from build123d import *

# Parameters (mm, degrees)
SKETCH1_W           = 129
SKETCH1_H           = 7
BOSS_EXTRUDE1_DEPTH = 7
BOSS_EXTRUDE2_START = 0.5
BOSS_EXTRUDE2_DEPTH = 0.5
SKETCH3_W           = 131
SKETCH3_H           = 7
CUT_EXTRUDE4_DEPTH  = 7
CUT_EXTRUDE5_DEPTH  = 7


with BuildPart() as part:
    # Sketch1 → Boss-Extrude1 (new body)
    with BuildSketch(Plane(origin=(0, 0, 0), x_dir=(1, 0, 0), z_dir=(0, 1, 0))):
        with BuildLine():
            Line((-65.5, 5.5), (-65.5, -3.5))
            ThreePointArc((-65.5, -3.5), (0, -56.5), (65.5, -3.5))
            Line((65.5, -3.5), (65.5, 5.5))
            Line((65.5, 5.5), (-65.5, 5.5))
        make_face()
        Rectangle(SKETCH1_W, SKETCH1_H, mode=Mode.SUBTRACT)
    extrude(amount=BOSS_EXTRUDE1_DEPTH)

    # Sketch2 → Boss-Extrude2 (add)
    with BuildSketch(Plane.XZ.offset(BOSS_EXTRUDE2_START)):
        with BuildLine():
            Line((-65.5, -5.5), (65.5, -5.5))
            Line((65.5, -5.5), (65.5, 3.5))
            ThreePointArc((65.5, 3.5), (0, 56.5), (-65.5, 3.5))
            Line((-65.5, 3.5), (-65.5, -5.5))
        make_face()
    extrude(amount=-BOSS_EXTRUDE2_DEPTH)

    # Sketch3 → Cut-Extrude4 (cut)
    with BuildSketch(Plane(origin=(0, 7, 0), x_dir=(1, 0, 0), z_dir=(0, 1, 0))):
        Rectangle(SKETCH3_W, SKETCH3_H)
    extrude(amount=-CUT_EXTRUDE4_DEPTH, mode=Mode.SUBTRACT)

    # Sketch4 → Cut-Extrude5 (cut)
    with BuildSketch(Plane(origin=(0, 7, 0), x_dir=(1, 0, 0), z_dir=(0, 1, 0))):
        with BuildLine():
            Line((58.998041221, -8.5), (-58.998041221, -8.5))
            ThreePointArc((-58.998041221, -8.5), (0, -51.5), (58.998041221, -8.5))
        make_face()
    extrude(amount=-CUT_EXTRUDE5_DEPTH, mode=Mode.SUBTRACT)


solid = part.part
Design review of the part built by this model. Coordinates are the model's own, in mm. A direction names the side the tool comes from. Give positions to 0.01 mm unless a question says otherwise; leave off trailing zeros. Loops run counter-clockwise (first coordinate to the right, second up) from the corner with the lowest first, then second, coordinate; pieces in that order, holes last. Notation, with made-up numbers: (38, 72.5) - (80, 72.5) arc R22 ccw to (80, 82.5) - close; hole circle Ø6 at (-30.75, 86). An arc over 180 degrees is marked (long way). Write item = value, one per line.
1) Tool access review of faces 5 (the face through (65.5, 3, -4)), 6 (the face through (1, 4, 8.5)), 7 (the face through (-1, 4, -3.5)): name each direction out of +Z, -Z, +X, -X, +Y, -Y from which nothing blocks a thin tool from reaching the whole face with its end or side.
Result sheet:
face_5 = +Z, -Z, +X, +Y, -Y
face_6 = +Y
face_7 = +X, -X, +Y
2) Take a section at A-A on y = 4. State the section outline as (x, z) points.
Result sheet:
outline = (-65.5, -5.5) - (65.5, -5.5) - (65.5, -3.5) - (-65.5, -3.5) - close; (-65.5, 3.5) - (65.5, 3.5) arc R66.97 ccw to start; hole (-59, 8.5) - (59, 8.5) arc R61.97 ccw to start
3) Take a section at D-D on x = -41.5. State the section outline as (y, z) points, and give its area (3 significant figures).
Result sheet:
outline = (-0.5, -5.5) - (7, -5.5) - (7, -3.5) - (0, -3.5) - (0, 3.5) - (7, 3.5) - (7, 8.5) - (0, 8.5) - (0, 35.55) - (7, 35.55) - (7, 42.09) - (-0.5, 42.09) - close
area = 119 mm2
4) Clearance check with flat-ended pins moving along their axes: pin 1 Ø1.5 at (x, y) = (48, 4) entering from +Z; pin 2 Ø1.5 at (y, z) = (5, 13) entering from +X; pin 3 Ø1.5 at (y, z) = (5.5, 32.5) entering from +X. State where each tip first meets the part, or that it passes through.
Result sheet:
pin_1 = 36.99
pin_2 = 63
pin_3 = 51.99
5) Take a section at C-C on z = 26.5. State the section outline as (x, y) points.
Result sheet:
outline = (-55.84, -0.5) - (55.84, -0.5) - (55.84, 7) - (49.74, 7) - (49.74, 0) - (-49.74, 0) - (-49.74, 7) - (-55.84, 7) - close
6) To check wall thickness, follow line 1 (Z direction, x = 56, y = 2.5); line 2 (Z direction, x = 32, y = 5); line 3 (Y direction, x = -44, z = -2). State the ranges of each line that lie inside material, in increasing order.
Result sheet:
line_1 = -5.5 to -3.5, 3.5 to 8.5, 16.07 to 26.26
line_2 = -5.5 to -3.5, 3.5 to 8.5, 42.6 to 48.36
line_3 = -0.5 to 0
7) Take a section at B-B on x = 47. State the section outline as (y, z) points.
Result sheet:
outline = (-0.5, -5.5) - (7, -5.5) - (7, -3.5) - (0, -3.5) - (0, 3.5) - (7, 3.5) - (7, 8.5) - (0, 8.5) - (0, 29.92) - (7, 29.92) - (7, 37.24) - (-0.5, 37.24) - close
8) Draft analysis for pull direction Z (two halves, no side actions). For faces 1 (the face through (-1, 0, 25)), 2 (the face through (1.276, 3.198, 56.488)), 3 (the face through (-1, -0.5, 19)), 4 (the face through (-1, 3, -5.5)), state which applies: +Z half, -Z half, draft (parallel to the pull), parting line (faces both ways), or undercut.
Result sheet:
face_1 = undercut
face_2 = +Z half
face_3 = draft
face_4 = -Z half
